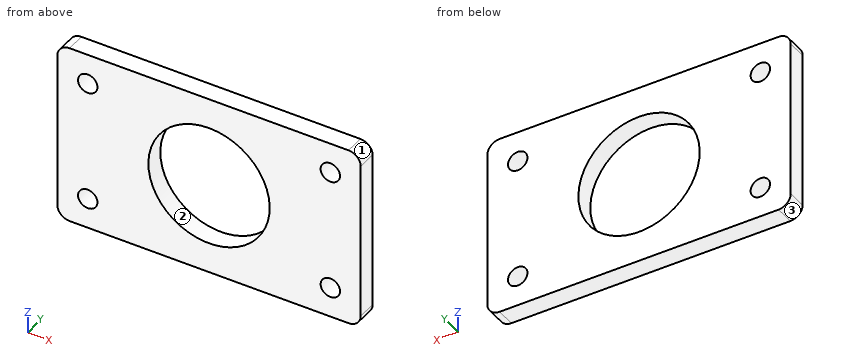
from build123d import *

# Parameters (mm, degrees)
SKETCH1_W                = 50
SKETCH1_H                = 30
SKETCH1_R                = 10
BOSS_EXTRUDE1_DEPTH      = 3.175
M3_CLEARANCE_HOLE1_D     = 3.2
M3_CLEARANCE_HOLE1_DEPTH = 3.175
FILLET1_R                = 2


with BuildPart() as part:
    # Sketch1 → Boss-Extrude1 (new body)
    with BuildSketch(Plane(origin=(0, 0, 0), x_dir=(1, 0, 0), z_dir=(0, 1, 0))):
        Rectangle(SKETCH1_W, SKETCH1_H)
        with Locations(Location((0, 0, 0), (0, 0, 270))):
            Circle(SKETCH1_R, mode=Mode.SUBTRACT)
    extrude(amount=BOSS_EXTRUDE1_DEPTH)

    # M3 Clearance Hole1
    with Locations(Plane(origin=(0, 3.175, 0), x_dir=(1, 0, 0), z_dir=(0, 1, 0))):
        with Locations((0, 0), (-20, 10), (20, -10), (20, 10), (-20, -10)):
            Hole(M3_CLEARANCE_HOLE1_D / 2, depth=M3_CLEARANCE_HOLE1_DEPTH)

    # Fillet1
    fillet1_edges = [part.edges().sort_by_distance(p)[0] for p in [
        (-25, 1.5875, -15),
        (25, 1.5875, -15),
        (25, 1.5875, 15),
        (-25, 1.5875, 15),
    ]]
    fillet(fillet1_edges, radius=FILLET1_R)


solid = part.part
Could you check a few things on this model? Use its own coordinates, in mm. Face numbers are marked on the shaded views. Give positions to 0.01 mm unless a question says otherwise; leave off trailing zeros. Order: outer loops, then holes, each group sorted by start corner. A loop starts at its lowest first (then second) coordinate and runs counter-clockwise, first axis right, second up. Notation, with made-up numbers: (17.25, 7) - (74.25, 7) arc R21 cw to (74.25, 38) - close; hole circle Ø10 at (83, 87). An arc over 180 degrees is marked (long way). One line per item, written item: value. Start each with the question number.
1. Imagine slicing it at C-C on x = 0.5. List the corners of the cut face in (y, z) for me (1 decimal).
2. Imagine slicing it at B-B on z = 0. List the corners of the cut face in (x, y) for me (3 decimals).
3. Imagine slicing it at A-A on x = 20. List the corners of the cut face in (y, z) for me (3 decimals).
4. Imagine slicing it at D-D on y = 0.5. List the corners of the cut face in (x, z) for me, plus the area to 3 significant figures.
5. Thinking about a two-plate mould opening in X: for the marked faces 1, 2 and 3, which applies, +X half, -X half, draft (parallel to the pull), parting line (faces both ways), or undercut?
6. If I drill on probe 1 along Z at (x, y) = (-20, 1.8); probe 2 along X at (y, z) = (1.2, 0); probe 3 along X at (y, z) = (0.95, 9), over which ranges is the centre line in solid material (lowest first)?
Values:
1. outline: (0, -15) - (3.2, -15) - (3.2, -10) - (0, -10) - close; (0, 10) - (3.2, 10) - (3.2, 15) - (0, 15) - close
2. outline: (-25, 0) - (-10, 0) - (-10, 3.175) - (-25, 3.175) - close; (10, 0) - (25, 0) - (25, 3.175) - (10, 3.175) - close
3. outline: (0, -15) - (3.175, -15) - (3.175, -11.6) - (0, -11.6) - close; (0, -8.4) - (3.175, -8.4) - (3.175, 8.4) - (0, 8.4) - close; (0, 11.6) - (3.175, 11.6) - (3.175, 15) - (0, 15) - close
4. outline: (-25, -13) arc R2 ccw to (-23, -15) - (23, -15) arc R2 ccw to (25, -13) - (25, 13) arc R2 ccw to (23, 15) - (-23, 15) arc R2 ccw to (-25, 13) - close; hole circle Ø3.2 at (-20, -10); hole circle Ø3.2 at (-20, 10); hole circle Ø20 at (0, 0); hole circle Ø3.2 at (20, -10); hole circle Ø3.2 at (20, 10)
4. area: 1,150 mm²
5. face 1: +X half
5. face 2: undercut
5. face 3: -X half
6. probe 1: -15 to -11.6, -8.4 to 8.4, 11.6 to 15
6. probe 2: -25 to -10, 10 to 25
6. probe 3: -25 to -21.25, -18.75 to -4.36, 4.36 to 18.75, 21.25 to 25
